Source: CAD feature listing. Evaluate the final solid. Frame: model axes, mm. Give positions to 0.01 mm unless a question says otherwise; leave off trailing zeros. Loops run counter-clockwise (first coordinate to the right, second up) from the corner with the lowest first, then second, coordinate; pieces in that order, holes last.
```python
from build123d import *

# Parameters (mm, degrees)
SKETCH1_W           = 150
SKETCH1_H           = 200
BOSS_EXTRUDE1_DEPTH = 10
SKETCH2_R           = 2.5
SKETCH2_R_2         = 2.75
CUT_EXTRUDE1_DEPTH  = 11


with BuildPart() as part:
    # Sketch1 → Boss-Extrude1 (new body)
    with BuildSketch(Plane(origin=(0, 0, 0), x_dir=(1, 0, 0), z_dir=(0, 1, 0))):
        Rectangle(SKETCH1_W, SKETCH1_H)
    extrude(amount=BOSS_EXTRUDE1_DEPTH)

    # Sketch2 → Cut-Extrude1 (cut, through all)
    with BuildSketch(Plane.XZ):
        with Locations((-70, 93)):
            Circle(SKETCH2_R)
        with Locations((-30, 93)):
            Circle(SKETCH2_R)
        with Locations((-30, 53)):
            Circle(SKETCH2_R)
        with Locations((-70, 53)):
            Circle(SKETCH2_R)
        with Locations((70, 53)):
            Circle(SKETCH2_R)
        with Locations((30, 53)):
            Circle(SKETCH2_R)
        with Locations((30, 93)):
            Circle(SKETCH2_R)
        with Locations((70, 93)):
            Circle(SKETCH2_R)
        with Locations((-70, -9)):
            Circle(SKETCH2_R)
        with Locations((-30, -9)):
            Circle(SKETCH2_R)
        with Locations((-30, -49)):
            Circle(SKETCH2_R)
        with Locations((-70, -49)):
            Circle(SKETCH2_R)
        with Locations((70, -49)):
            Circle(SKETCH2_R)
        with Locations((30, -49)):
            Circle(SKETCH2_R)
        with Locations((30, -9)):
            Circle(SKETCH2_R)
        with Locations((70, -9)):
            Circle(SKETCH2_R)
        with Locations((-23, 90)):
            Circle(SKETCH2_R_2)
        with Locations((23, 90)):
            Circle(SKETCH2_R_2)
    extrude(amount=-CUT_EXTRUDE1_DEPTH, mode=Mode.SUBTRACT)


solid = part.part
```
(1) Section B-B, the plane z = -49. Return the cut outline in (x, y).
A:
outline: (-75, 0) - (-72.5, 0) - (-72.5, 10) - (-75, 10) - close; (-67.5, 0) - (-32.5, 0) - (-32.5, 10) - (-67.5, 10) - close; (-27.5, 0) - (27.5, 0) - (27.5, 10) - (-27.5, 10) - close; (32.5, 0) - (67.5, 0) - (67.5, 10) - (32.5, 10) - close; (72.5, 0) - (75, 0) - (75, 10) - (72.5, 10) - close
(2) Section A-A, the plane x = 23. Return the cut outline in (y, z).
A:
outline: (0, -100) - (10, -100) - (10, 87.25) - (0, 87.25) - close; (0, 92.75) - (10, 92.75) - (10, 100) - (0, 100) - close
(3) Ray query, line 1 along Z through (x, y) = (-70, 3); line 2 along Z through (x, y) = (-29.5, 1.5); line 3 along Z through (x, y) = (-24, 9.25). Return the intervals inside material, ascending.
A:
line 1: z = -100 to -51.5, -46.5 to -11.5, -6.5 to 50.5, 55.5 to 90.5, 95.5 to 100
line 2: z = -100 to -51.45, -46.55 to -11.45, -6.55 to 50.55, 55.45 to 90.55, 95.45 to 100
line 3: z = -100 to 87.44, 92.56 to 100
(4) Mould query, pull axis X, two halves, no side actions, for faces 1 (the flat face through (75, 5, 1)), 2 (the cylindrical face through (-72, 4.9, -10.5)), 3 (the flat face through (-1, 0, -1)). Classes: pulls with the +X half, pulls with the -X half, needs draft (parallel to the pull), parting line crosses it, or undercut.
A:
face 1: pulls with the +X half
face 2: undercut
face 3: needs draft
(5) Section C-C, the plane x = 70. Return the cut outline in (y, z).
A:
outline: (0, -100) - (10, -100) - (10, -51.5) - (0, -51.5) - close; (0, -46.5) - (10, -46.5) - (10, -11.5) - (0, -11.5) - close; (0, -6.5) - (10, -6.5) - (10, 50.5) - (0, 50.5) - close; (0, 55.5) - (10, 55.5) - (10, 90.5) - (0, 90.5) - close; (0, 95.5) - (10, 95.5) - (10, 100) - (0, 100) - close
